Design review of the part built by this model. Coordinates are the model's own, in mm. Face numbers are marked on the shaded views. A direction names the side the tool comes from. Give positions to 0.01 mm unless a question says otherwise; leave off trailing zeros. Write each loop counter-clockwise with the first axis right and the second up, starting at its lowest first coordinate (ties: lowest second). Pieces come first, ordered by that corner, then holes. Notation, with made-up numbers: M 60.5,78 L 80.5,78 A23 ccw 80.5,94 Z; hole C -32.75,20.5 d9. An arc over 180 degrees is marked long. One line per item, written item: value. Start each with the question number.
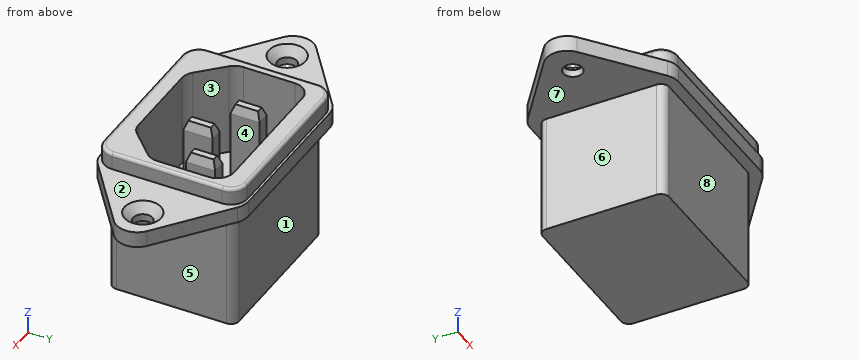
```python
from build123d import *

# Parameters (mm, degrees)
EXTRUDE1_DEPTH                                    = 5.15
FILLET1_R                                         = 1
EXTRUDE2_DEPTH                                    = 17.78
EXTRUDE3_DEPTH                                    = 13.97
EXTRUDE4_DEPTH                                    = 3.81
FILLET2_R                                         = 2.5
SKETCH5_W                                         = 2
SKETCH5_H                                         = 4.4
EXTRUDE5_DEPTH                                    = 12.7
CHAMFER1_SIZE                                     = 0.5
CHAMFER1_SIZE2                                    = 1.37373871
CHAMFER1_PART_2_SIZE                              = 0.5
CHAMFER1_PART_2_SIZE2                             = 1.37373871
CHAMFER1_PART_3_SIZE                              = 0.5
CHAMFER1_PART_3_SIZE2                             = 1.37373871
CHAMFER2_SIZE                                     = 0.5
CHAMFER2_SIZE2                                    = 1.37373871
CHAMFER2_PART_2_SIZE                              = 0.5
CHAMFER2_PART_2_SIZE2                             = 1.37373871
CHAMFER2_PART_3_SIZE                              = 0.5
CHAMFER2_PART_3_SIZE2                             = 1.37373871
FILLET3_R                                         = 0.5
SKETCH10_OUTSIDE_W                                = 57.448
SKETCH10_OUTSIDE_H                                = 47.956
EXTRUDE10_DEPTH                                   = 20.12
SKETCH11_OUTSIDE_W                                = 37.296
SKETCH11_OUTSIDE_H                                = 31.886
EXTRUDE11_DEPTH                                   = 21.39
EXTRUDE12_DEPTH                                   = 2.413
CSK_FOR_M2_5_FLAT_HEAD_MACHINE_SCREW1_D           = 2.9
CSK_FOR_M2_5_FLAT_HEAD_MACHINE_SCREW1_CSINK_D     = 5.5
CSK_FOR_M2_5_FLAT_HEAD_MACHINE_SCREW1_CSINK_ANGLE = 90


with BuildPart() as part:
    # Sketch1 → Extrude1 (new body)
    with BuildSketch(Plane.XY):
        with BuildLine():
            Line((-13.6, 17), (13.6, 17))
            Line((13.6, 17), (21.429179607, 1.341640786))
            ThreePointArc((21.429179607, 1.341640786), (21.745898034, 0), (21.429179607, -1.341640786))
            Line((21.429179607, -1.341640786), (13.6, -17))
            Line((13.6, -17), (-13.6, -17))
            Line((-13.6, -17), (-21.429179607, -1.341640786))
            ThreePointArc((-21.429179607, -1.341640786), (-21.745898034, 0), (-21.429179607, 1.341640786))
            Line((-21.429179607, 1.341640786), (-13.6, 17))
        make_face()
    extrude(amount=-EXTRUDE1_DEPTH)

    # Fillet1
    fillet1_edges = [part.edges().sort_by_distance(p)[0] for p in [
        (-13.6, 17, -2.575),
        (13.6, 17, -2.575),
        (13.6, -17, -2.575),
        (-13.6, -17, -2.575),
    ]]
    fillet(fillet1_edges, radius=FILLET1_R)

    # Sketch2 → Extrude2 (add)
    with BuildSketch(Plane(origin=(0, 0, -5.15), x_dir=(-1, 0, 0), z_dir=(0, 0, -1))):
        with BuildLine():
            Line((-12.9, 15.65), (12.9, 15.65))
            ThreePointArc((12.9, 15.65), (13.607106781, 15.357106781), (13.9, 14.65))
            Line((13.9, 14.65), (13.9, -14.65))
            ThreePointArc((13.9, -14.65), (13.607106781, -15.357106781), (12.9, -15.65))
            Line((12.9, -15.65), (-12.9, -15.65))
            ThreePointArc((-12.9, -15.65), (-13.607106781, -15.357106781), (-13.9, -14.65))
            Line((-13.9, -14.65), (-13.9, 14.65))
            ThreePointArc((-13.9, 14.65), (-13.607106781, 15.357106781), (-12.9, 15.65))
        make_face()
    extrude(amount=EXTRUDE2_DEPTH)

    # Sketch3 → Extrude3 (cut)
    with BuildSketch(Plane.XY):
        Polygon((-12.15, -9.18), (-7.15, -14.18), (7.15, -14.18), (12.15, -9.18), (12.15, 2.12), (-12.15, 2.12), align=None)
    extrude(amount=-EXTRUDE3_DEPTH, mode=Mode.SUBTRACT)

    # Sketch4 → Extrude4 (cut)
    with BuildSketch(Plane.XY):
        with BuildLine():
            Line((-21.429179607, -1.341640786), (-13.876393202, -16.447213595))
            ThreePointArc((-13.876393202, -16.447213595), (-13.507697123, -16.850650808), (-12.981966011, -17))
            Line((-12.981966011, -17), (12.981966011, -17))
            ThreePointArc((12.981966011, -17), (13.507697123, -16.850650808), (13.876393202, -16.447213595))
            Line((13.876393202, -16.447213595), (21.429179607, -1.341640786))
            ThreePointArc((21.429179607, -1.341640786), (21.745898034, 0), (21.429179607, 1.341640786))
            Line((21.429179607, 1.341640786), (13.876393202, 16.447213595))
            ThreePointArc((13.876393202, 16.447213595), (13.507697123, 16.850650808), (12.981966011, 17))
            Line((12.981966011, 17), (-12.981966011, 17))
            ThreePointArc((-12.981966011, 17), (-13.507697123, 16.850650808), (-13.876393202, 16.447213595))
            Line((-13.876393202, 16.447213595), (-21.429179607, 1.341640786))
            ThreePointArc((-21.429179607, 1.341640786), (-21.745898034, 0), (-21.429179607, -1.341640786))
        make_face()
        with BuildLine():
            Line((-11, 4.8886), (11, 4.8886))
            ThreePointArc((11, 4.8886), (12.767766953, 4.156366953), (13.5, 2.3886))
            Line((13.5, 2.3886), (13.5, -14.2014))
            ThreePointArc((13.5, -14.2014), (12.767766953, -15.969166953), (11, -16.7014))
            Line((11, -16.7014), (-11, -16.7014))
            ThreePointArc((-11, -16.7014), (-12.767766953, -15.969166953), (-13.5, -14.2014))
            Line((-13.5, -14.2014), (-13.5, 2.3886))
            ThreePointArc((-13.5, 2.3886), (-12.767766953, 4.156366953), (-11, 4.8886))
        make_face(mode=Mode.SUBTRACT)
    extrude(amount=-EXTRUDE4_DEPTH, mode=Mode.SUBTRACT)

    # Fillet2
    fillet2_edges = [part.edges().sort_by_distance(p)[0] for p in [
        (-12.15, -9.18, -6.985),
        (-12.15, 2.12, -6.985),
        (12.15, 2.12, -6.985),
        (12.15, -9.18, -6.985),
        (7.15, -14.18, -6.985),
        (-7.15, -14.18, -6.985),
    ]]
    fillet(fillet2_edges, radius=FILLET2_R)

    # Sketch5 → Extrude5 (add)
    with BuildSketch(Plane.XY.offset(-13.97)):
        with Locations((-6.25, -4.2)):
            Rectangle(SKETCH5_W, SKETCH5_H)
        with Locations((0, -7.95)):
            Rectangle(SKETCH5_W, SKETCH5_H)
        with Locations((6.25, -4.2)):
            Rectangle(SKETCH5_W, SKETCH5_H)
    extrude(amount=EXTRUDE5_DEPTH)

    # Chamfer1
    chamfer1_edges = [part.edges().sort_by_distance(p)[0] for p in [
        (-6.25, -6.4, -1.27),
        (-6.25, -2, -1.27),
    ]]
    chamfer1_side = [part.faces().sort_by_distance(p)[0] for p in [
        (-6.25, -4.2, -1.27),
    ]]
    chamfer(chamfer1_edges, length=CHAMFER1_SIZE, length2=CHAMFER1_SIZE2, reference=chamfer1_side[0])

    # Chamfer1 part 2
    chamfer1_part_2_edges = [part.edges().sort_by_distance(p)[0] for p in [
        (0, -10.15, -1.27),
        (0, -5.75, -1.27),
    ]]
    chamfer1_part_2_side = [part.faces().sort_by_distance(p)[0] for p in [
        (0, -7.95, -1.27),
    ]]
    chamfer(chamfer1_part_2_edges, length=CHAMFER1_PART_2_SIZE, length2=CHAMFER1_PART_2_SIZE2, reference=chamfer1_part_2_side[0])

    # Chamfer1 part 3
    chamfer1_part_3_edges = [part.edges().sort_by_distance(p)[0] for p in [
        (6.25, -2, -1.27),
        (6.25, -6.4, -1.27),
    ]]
    chamfer1_part_3_side = [part.faces().sort_by_distance(p)[0] for p in [
        (6.25, -4.2, -1.27),
    ]]
    chamfer(chamfer1_part_3_edges, length=CHAMFER1_PART_3_SIZE, length2=CHAMFER1_PART_3_SIZE2, reference=chamfer1_part_3_side[0])

    # Chamfer2
    chamfer2_edges = [part.edges().sort_by_distance(p)[0] for p in [
        (7.25, -4.2, -1.27),
        (5.25, -4.2, -1.27),
    ]]
    chamfer2_side = [part.faces().sort_by_distance(p)[0] for p in [
        (6.25, -4.2, -1.27),
    ]]
    chamfer(chamfer2_edges, length=CHAMFER2_SIZE, length2=CHAMFER2_SIZE2, reference=chamfer2_side[0])

    # Chamfer2 part 2
    chamfer2_part_2_edges = [part.edges().sort_by_distance(p)[0] for p in [
        (1, -7.95, -1.27),
        (-1, -7.95, -1.27),
    ]]
    chamfer2_part_2_side = [part.faces().sort_by_distance(p)[0] for p in [
        (0, -7.95, -1.27),
    ]]
    chamfer(chamfer2_part_2_edges, length=CHAMFER2_PART_2_SIZE, length2=CHAMFER2_PART_2_SIZE2, reference=chamfer2_part_2_side[0])

    # Chamfer2 part 3
    chamfer2_part_3_edges = [part.edges().sort_by_distance(p)[0] for p in [
        (-7.25, -4.2, -1.27),
        (-5.25, -4.2, -1.27),
    ]]
    chamfer2_part_3_side = [part.faces().sort_by_distance(p)[0] for p in [
        (-6.25, -4.2, -1.27),
    ]]
    chamfer(chamfer2_part_3_edges, length=CHAMFER2_PART_3_SIZE, length2=CHAMFER2_PART_3_SIZE2, reference=chamfer2_part_3_side[0])

    # Fillet3
    fillet3_edges = [part.edges().sort_by_distance(p)[0] for p in [
        (-12.767766953, 4.156366953, 0),
        (0, 4.8886, 0),
        (12.767766953, 4.156366953, 0),
        (13.5, -5.9064, 0),
        (12.767766953, -15.969166953, 0),
        (0, -16.7014, 0),
        (-12.767766953, -15.969166953, 0),
        (-13.5, -5.9064, 0),
    ]]
    fillet(fillet3_edges, radius=FILLET3_R)

    # Sketch10 outside → Extrude10 (cut, through all)
    with BuildSketch(Plane.XY.offset(-3.81)):
        Rectangle(SKETCH10_OUTSIDE_W, SKETCH10_OUTSIDE_H)
        with BuildLine():
            Line((-13.5, 2.3886), (-13.5, -14.2014))
            ThreePointArc((-13.5, -14.2014), (-12.767766953, -15.969166953), (-11, -16.7014))
            Line((-11, -16.7014), (11, -16.7014))
            ThreePointArc((11, -16.7014), (12.767766953, -15.969166953), (13.5, -14.2014))
            Line((13.5, -14.2014), (13.5, 2.3886))
            ThreePointArc((13.5, 2.3886), (12.767766953, 4.156366953), (11, 4.8886))
            Line((11, 4.8886), (-11, 4.8886))
            ThreePointArc((-11, 4.8886), (-12.767766953, 4.156366953), (-13.5, 2.3886))
        make_face(mode=Mode.SUBTRACT)
    extrude(amount=-EXTRUDE10_DEPTH, mode=Mode.SUBTRACT)

    # Sketch11 outside → Extrude11 (cut, through all)
    with BuildSketch(Plane.XY.offset(-2.54)):
        with Locations((0, -5.906)):
            Rectangle(SKETCH11_OUTSIDE_W, SKETCH11_OUTSIDE_H)
        with BuildLine():
            Line((-11, -15.4314), (11, -15.4314))
            ThreePointArc((11, -15.4314), (11.869741341, -15.071141341), (12.23, -14.2014))
            Line((12.23, -14.2014), (12.23, 2.3886))
            ThreePointArc((12.23, 2.3886), (11.869741341, 3.258341341), (11, 3.6186))
            Line((11, 3.6186), (-11, 3.6186))
            ThreePointArc((-11, 3.6186), (-11.869741341, 3.258341341), (-12.23, 2.3886))
            Line((-12.23, 2.3886), (-12.23, -14.2014))
            ThreePointArc((-12.23, -14.2014), (-11.869741341, -15.071141341), (-11, -15.4314))
        make_face(mode=Mode.SUBTRACT)
    extrude(amount=-EXTRUDE11_DEPTH, mode=Mode.SUBTRACT)

    # Sketch12 → Extrude12 (add)
    with BuildSketch(Plane(origin=(0, 0, -2.54), x_dir=(-1, 0, 0), z_dir=(0, 0, -1))):
        with BuildLine():
            Line((-11.43, 5.2696), (11.43, 5.2696))
            ThreePointArc((11.43, 5.2696), (12.451483532, 5.100793007), (13.364347496, 4.612322138))
            Line((13.364347496, 4.612322138), (23.778347496, -3.388677862))
            ThreePointArc((23.778347496, -3.388677862), (25.019, -5.9064), (23.778347496, -8.424122138))
            Line((23.778347496, -8.424122138), (13.364347496, -16.425122138))
            ThreePointArc((13.364347496, -16.425122138), (12.451483532, -16.913593007), (11.43, -17.0824))
            Line((11.43, -17.0824), (-11.43, -17.0824))
            ThreePointArc((-11.43, -17.0824), (-12.451483532, -16.913593007), (-13.364347496, -16.425122138))
            Line((-13.364347496, -16.425122138), (-23.778347496, -8.424122138))
            ThreePointArc((-23.778347496, -8.424122138), (-25.019, -5.9064), (-23.778347496, -3.388677862))
            Line((-23.778347496, -3.388677862), (-13.364347496, 4.612322138))
            ThreePointArc((-13.364347496, 4.612322138), (-12.451483532, 5.100793007), (-11.43, 5.2696))
        make_face()
        with BuildLine():
            Line((12.23, 2.3886), (12.23, -14.2014))
            ThreePointArc((12.23, -14.2014), (11.869741341, -15.071141341), (11, -15.4314))
            Line((11, -15.4314), (-11, -15.4314))
            ThreePointArc((-11, -15.4314), (-11.869741341, -15.071141341), (-12.23, -14.2014))
            Line((-12.23, -14.2014), (-12.23, 2.3886))
            ThreePointArc((-12.23, 2.3886), (-11.869741341, 3.258341341), (-11, 3.6186))
            Line((-11, 3.6186), (11, 3.6186))
            ThreePointArc((11, 3.6186), (11.869741341, 3.258341341), (12.23, 2.3886))
        make_face(mode=Mode.SUBTRACT)
    extrude(amount=EXTRUDE12_DEPTH)

    # CSK for M2.5 Flat Head Machine Screw1 (through all)
    with Locations(Plane.XY.offset(-2.54)):
        with Locations((-20.32, -5.9064), (20.32, -5.9064)):
            CounterSinkHole(CSK_FOR_M2_5_FLAT_HEAD_MACHINE_SCREW1_D / 2, CSK_FOR_M2_5_FLAT_HEAD_MACHINE_SCREW1_CSINK_D / 2, counter_sink_angle=CSK_FOR_M2_5_FLAT_HEAD_MACHINE_SCREW1_CSINK_ANGLE)


solid = part.part
```
Q1. Take a section at B-B, the plane x = 8.5. Give the boundary of the cut face in (y, z).
Q2. Machinability: for the marked faces 4, 5, 6, 7 and 8, which of the approach directions +Z, -Z, +X, -X, +Y, -Y give a long, thin tool a straight path to every point of the face, cutting with its end or side? Answer none if there is none.
Q3. Take a section at A-A, the plane z = -10.75. State how many separate pieces and enclosed holes the cut face has, then the cut area to 3 significant figures.
Q4. Take a section at D-D, the plane x = -20.32. Give the boundary of the cut face in (y, z).
Q5. Take a section at C-C, the plane z = -14.5. Give the boundary of the cut face in (x, y).
Q6. The part is to be moulded in two halves that separate along Y. For the marked faces 1, 2 and 3, say which applies: pulls with the +Y half, pulls with the -Y half, needs draft (parallel to the pull), parting line crosses it, or undercut.
Q7. Wall thickness on line 1 (Y direction, x = -2.5, z = -8); line 2 (X direction, y = 1.5, z = -17.5); line 3 (Z direction, x = -15.5, y = -4.25): over which ranges is each line inside the solid? List them lowest first. Write a range as from..to.
Q8. For P1, Ø3.5, axis at y = -5.5, z = -8, coming from the +X side; P2, Ø4, axis at y = -2.5, z = -5.5, coming from the +X side; P3, Ø1.1, axis at x = 6, y = -4.5, coming from the +Z side, all flat-tipped, find the tip position at first contact; note any pin that passes through.
Results list:
1. outline: M -17.08,-4.95 L -15.43,-4.95 L -15.43,-22.93 L 3.62,-22.93 L 3.62,-4.95 L 5.27,-4.95 L 5.27,-2.54 L 4.89,-2.54 L 4.89,-0.5 A0.5 ccw 4.39,0 L 2.12,0 L 2.12,-13.97 L -12.83,-13.97 L -12.83,0 L -16.2,0 A0.5 ccw -16.7,-0.5 L -16.7,-2.54 L -17.08,-2.54 Z
2. face 4: +Z
2. face 5: -Z, +X, +Y, -Y
2. face 6: -Z, -X, +Y, -Y
2. face 7: -Z
2. face 8: -Z, +X, -X, -Y
3. separate pieces: 4
3. enclosed holes: 1
3. area: 123 mm^2
4. outline: M -11.08,-4.95 L -7.36,-4.95 L -7.36,-3.84 L -8.66,-2.54 L -11.08,-2.54 Z; M -4.46,-4.95 L -0.73,-4.95 L -0.73,-2.54 L -3.16,-2.54 L -4.46,-3.84 Z
5. outline: M -12.23,-14.2 A1.23 ccw -11,-15.43 L 11,-15.43 A1.23 ccw 12.23,-14.2 L 12.23,2.39 A1.23 ccw 11,3.62 L -11,3.62 A1.23 ccw -12.23,2.39 Z
6. face 1: pulls with the +Y half
6. face 2: needs draft
6. face 3: undercut
7. line 1: y = -15.43..-14.18, 2.12..3.62
7. line 2: x = -12.23..12.23
7. line 3: z = -4.95..-2.54
8. P1: stops at x = 12.23
8. P2: stops at x = 24.65
8. P3: stops at z = -1.27
